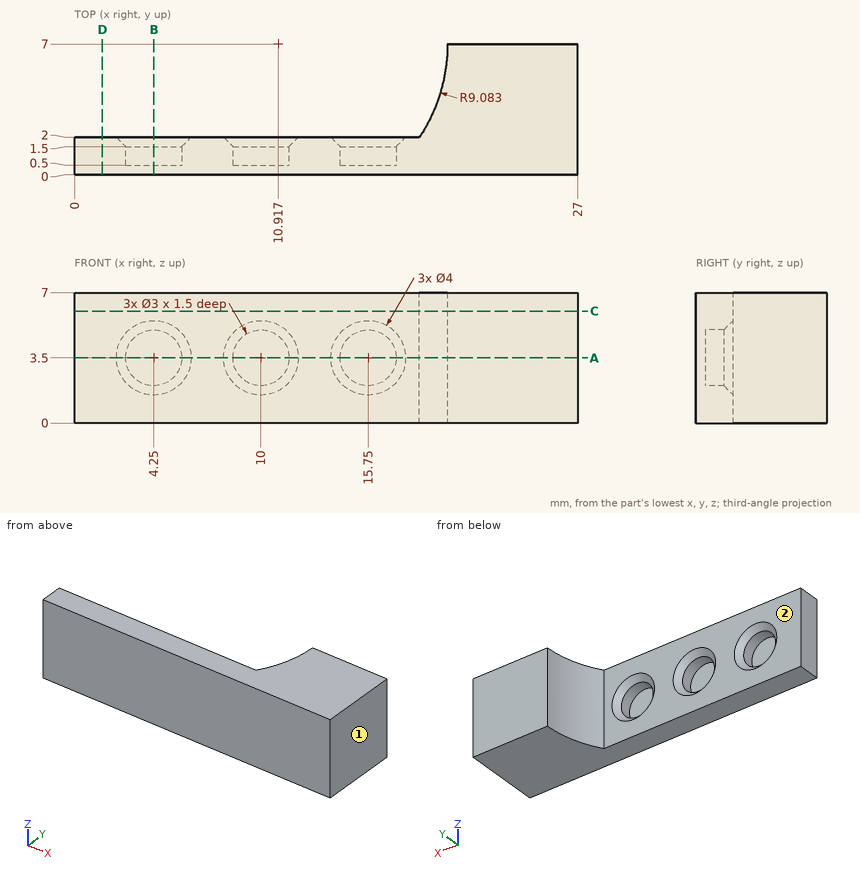
Could you check a few things on this drawing? It's one solid part, dimensions in mm from its lowest x, y, z. A direction names the side the tool comes from. Round coordinates to 2 decimals unless told otherwise and drop trailing zeros. Order: outer loops, then holes, each group sorted by start corner. A loop starts at its lowest first (then second) coordinate and runs counter-clockwise, first axis right, second up. Notation, with made-up numbers: M 67.5,-2 L 81.5,-2 A22 ccw 81.5,8 Z; hole C 45.25,80.5 d4. An arc over 180 degrees is marked long. One line per question, with ' | ' between items. Start each with the question number.
(1) Suppose I cut it at D-D on x = 1.5. List the corners of the cut face in (y, z) for me, then the cut area to 3 significant figures.
(2) Please list where these lines run through material, in increasing order: line 1 along Z through (x, y) = (10, 1.2); line 2 along Y through (x, z) = (17, 5.25); line 3 along X through (y, z) = (1, 2.25).
(3) Suppose I cut it at B-B on x = 4.25. List the corners of the cut face in (y, z) for me.
(4) For the marked faces 1 and 2, which set-ups out of +Z, -Z, +X, -X, +Y, -Y let a thin tool reach every point of the face, with its end or its side?
(5) Suppose I cut it at A-A on z = 3.5. List the corners of the cut face in (x, y) for me.
(6) For P1, Ø2.5, axis at x = 15.5, z = 4, coming from the +Y side; P2, Ø4, axis at x = 11, z = 1.5, coming from the +Y side, each with a flat end and sliding along its axis, tell me the tip position at first contact or that it passes through.
(7) Suppose I cut it at C-C on z = 6. List the corners of the cut face in (x, y) for me.
Geometry results:
1) outline: M 0,0 L 2,0 L 2,7 L 0,7 Z | area: 14.0 mm²
2) line 1: 0 to 2, 5 to 7 | line 2: 0 to 2 | line 3: 0 to 3.42, 5.08 to 9.17, 10.83 to 14.92, 16.58 to 27
3) outline: M 0,0 L 2,0 L 2,1.5 L 1.5,2 L 0.5,2 L 0.5,5 L 1.5,5 L 2,5.5 L 2,7 L 0,7 Z
4) face 1: +Z, -Z, +X, +Y, -Y | face 2: +Z, -Z, -X, +Y
5) outline: M 0,0 L 27,0 L 27,7 L 20,7 A9.08 cw 18.5,2 L 17.75,2 L 17.25,1.5 L 17.25,0.5 L 14.25,0.5 L 14.25,1.5 L 13.75,2 L 12,2 L 11.5,1.5 L 11.5,0.5 L 8.5,0.5 L 8.5,1.5 L 8,2 L 6.25,2 L 5.75,1.5 L 5.75,0.5 L 2.75,0.5 L 2.75,1.5 L 2.25,2 L 0,2 Z
6) P1: y = 1.81 | P2: y = 2
7) outline: M 0,0 L 27,0 L 27,7 L 20,7 A9.08 cw 18.5,2 L 0,2 Z
